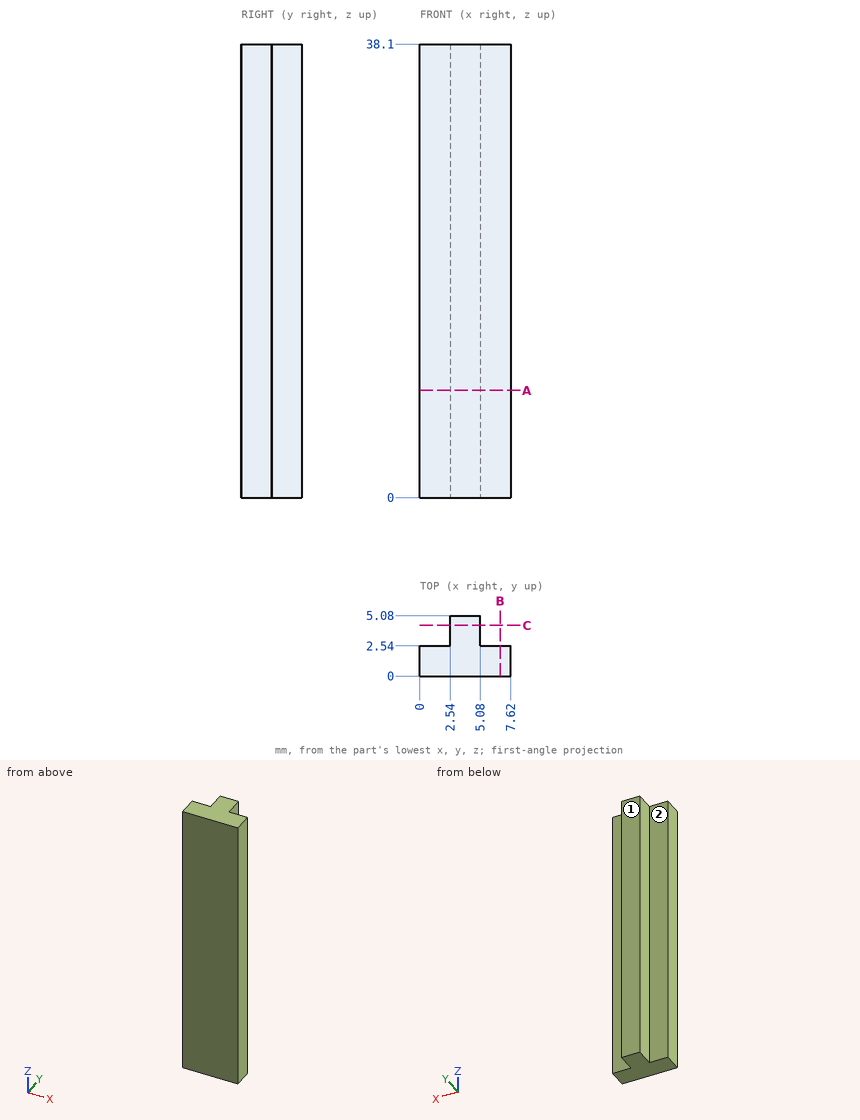
Part print with two shaded views. Sizes in mm from the minimum x, y, z corner. A direction names the side the tool comes from. Coordinates: 2 decimals unless noted, no trailing zeros. Write each loop counter-clockwise with the first axis right and the second up, starting at its lowest first coordinate (ties: lowest second). Pieces come first, ordered by that corner, then holes.
(1) 3-axis set-ups, long thin cutter, end or side, ignore diameter. For the marked faces 1 and 2: which of +Z, -Z, +X, -X, +Y, -Y reach the whole face in a straight line?
(2) Cut at A-A on z = 9. List the corners of the cut face in (x, y).
(3) Cut at B-B on x = 6.75. List the corners of the cut face in (y, z), and give its area (3 significant figures).
(4) Pin check, flat tips, straight feed: pin 1 Ø0.8 at (y, z) = (4, 23) entering from +X; pin 2 Ø1.3 at (x, z) = (6.5, 20.5) entering from +Y. Stop position of each tip, or through.
(5) Cut at C-C on y = 4.25. List the corners of the cut face in (x, z), and give its area (3 significant figures).
(6) Drill centre lines: line 1 (Y direction, x = 1, z = 11.5); line 2 (X direction, y = 4.4, z = 2.5). Where is each one in solid material? Low to high.
Working result:
1. face 1: +Z, -Z, +X, -X, +Y
1. face 2: +Z, -Z, -X, +Y
2. outline: (0, 0) - (7.62, 0) - (7.62, 2.54) - (5.08, 2.54) - (5.08, 5.08) - (2.54, 5.08) - (2.54, 2.54) - (0, 2.54) - close
3. outline: (0, 0) - (2.54, 0) - (2.54, 38.1) - (0, 38.1) - close
3. area: 96.8 mm2
4. pin 1: stops at x = 5.08
4. pin 2: stops at y = 2.54
5. outline: (2.54, 0) - (5.08, 0) - (5.08, 38.1) - (2.54, 38.1) - close
5. area: 96.8 mm2
6. line 1: y = 0 to 2.54
6. line 2: x = 2.54 to 5.08
